The listing builds one solid part. Answer for the finished solid, in the listing's coordinates (mm). A direction names the side the tool comes from. Round coordinates to 2 decimals unless told otherwise and drop trailing zeros. Write each loop counter-clockwise with the first axis right and the second up, starting at its lowest first coordinate (ties: lowest second). Pieces come first, ordered by that corner, then holes. Notation, with made-up numbers: (58, 41.25) - (117, 41.25) arc R9 cw to (117, 45.25) - close; hole circle Ø11 at (-38, 52.5). An arc over 180 degrees is marked (long way). Use a Markdown table: item, result. Add a question column.
1) Find the intervals of material crossed by probe 1 along X at (y, z) = (16.5, 0); probe 2 along Z at (x, y) = (0, 8); probe 3 along X at (y, z) = (-1, -7.5), in increasing order. Write a range as from..to.
2) A tool of negligible diameter and unlimited length cuts with its end or side. For faces 5 (the cylindrical face through (-74.77, -2.43, 0.08)), 6 (the flat face through (28, 50, 0)), 7 (the cylindrical face through (-3.905, 11.739, -0.867)), 8 (the flat face through (26, -5, 0)), 9 (the flat face through (1, -9.529, 0)), from which of +Z, -Z, +X, -X, +Y, -Y can it reach the whole face along a straight path? Write none if from no direction.
3) A cutting plane is placed at D-D (z = 0). State how many separate pieces and enclosed holes the cut face has, then the cut area to 3 significant figures.
4) Each of these flat-tipped pins is pushed along its axis until it touches: P1, Ø9, axis at x = -0.5, z = -1, coming from the +Y side; P2, Ø23, axis at x = 82.5, z = 11, coming from the +Y side; P3, Ø2, axis at x = 25, z = 5.5, coming from the +Y side. Where does it stop, or does it pass through?
5) A cutting plane is placed at C-C (y = 28.5). Give the vertices of the cut face in (x, z).
6) A cutting plane is placed at B-B (y = 9.5). Give the vertices of the cut face in (x, z).
7) A cutting plane is placed at A-A (x = -39). Give the vertices of the cut face in (y, z), then the cut area to 3 significant figures.
8) Determine the mould class of faces 1 (the flat face through (1, 17, -23)), 2 (the cylindrical face through (-90.474, -2.431, -0.087)), 3 (the cylindrical face through (-44.857, 29.877, -1.301)), 4 (the flat face through (-102.03, -2.63, 0.32)) for opening direction X: +X half, -X half, draft (parallel to the pull), parting line (faces both ways), or undercut.
```python
from build123d import *

# Parameters (mm, degrees)
BOSS_EXTRUDE1_DEPTH = 23
SKETCH2_R           = 6
CUT_EXTRUDE1_DEPTH  = 127.368508735
CUT_EXTRUDE2_DEPTH  = 54
CUT_EXTRUDE3_DEPTH  = 120.419428905
SKETCH5_R           = 4
CUT_EXTRUDE18_DEPTH = 24
SKETCH6_W           = 26
SKETCH6_H           = 26
CUT_EXTRUDE19_DEPTH = 10


with BuildPart() as part:
    # Sketch1 → Boss-Extrude1 (new, symmetric)
    with BuildSketch(Plane.XY):
        with BuildLine():
            Line((100, 4.470588235), (104, -9.529411765))
            Line((104, -9.529411765), (-104, -9.529411765))
            Line((-104, -9.529411765), (-100, 4.470588235))
            Line((-100, 4.470588235), (-54, 4.470588235))
            Line((-54, 4.470588235), (-54, 58.470588235))
            Line((-54, 58.470588235), (-28, 58.470588235))
            Line((-28, 58.470588235), (-28, 42.470588235))
            Line((-28, 42.470588235), (-24, 42.470588235))
            ThreePointArc((-24, 42.470588235), (0, 18.470588235), (24, 42.470588235))
            Line((24, 42.470588235), (28, 42.470588235))
            Line((28, 42.470588235), (28, 58.470588235))
            Line((28, 58.470588235), (54, 58.470588235))
            Line((54, 58.470588235), (54, 4.470588235))
            Line((54, 4.470588235), (100, 4.470588235))
        make_face()
    extrude(amount=BOSS_EXTRUDE1_DEPTH, both=True)

    # Sketch2 → Cut-Extrude1 (cut, through all)
    with BuildSketch(Plane(origin=(0, 58.470588235, 0), x_dir=(1, 0, 0), z_dir=(0, 1, 0))):
        with Locations(Location((-39, 0, 0), (0, 0, 270))):
            Circle(SKETCH2_R)
        with Locations(Location((39, 0, 0), (0, 0, 270))):
            Circle(SKETCH2_R)
    extrude(amount=-CUT_EXTRUDE1_DEPTH, mode=Mode.SUBTRACT)

    # Sketch3 → Cut-Extrude2 (cut)
    with BuildSketch(Plane(origin=(0, 58.470588235, 0), x_dir=(1, 0, 0), z_dir=(0, 1, 0))):
        with BuildLine():
            Line((-48.856934001, 23), (-69.801648505, 23))
            Line((-69.801648505, 23), (-69.801648505, -23))
            Line((-69.801648505, -23), (-48.856934001, -23))
            ThreePointArc((-48.856934001, -23), (-54, 0), (-48.856934001, 23))
        make_face()
        with BuildLine():
            Line((69.801648505, -23), (48.856934001, -23))
            ThreePointArc((48.856934001, -23), (54, 0), (48.856934001, 23))
            Line((48.856934001, 23), (69.801648505, 23))
            Line((69.801648505, 23), (69.801648505, -23))
        make_face()
    extrude(amount=-CUT_EXTRUDE2_DEPTH, mode=Mode.SUBTRACT)

    # Sketch4 → Cut-Extrude3 (cut, through all)
    with BuildSketch(Plane(origin=(0, 4.470588235, 0), x_dir=(1, 0, 0), z_dir=(0, 1, 0))):
        with BuildLine():
            Line((-86.259028478, 3.967568831), (-86.5, 3.974879835))
            ThreePointArc((-86.5, 3.974879835), (-90.474879835, 0), (-86.5, -3.974879835))
            Line((-86.5, -3.974879835), (-86.259028478, -3.967568831))
            Line((-86.259028478, -3.967568831), (-78.5, -3.732162222))
            ThreePointArc((-78.5, -3.732162222), (-74.767837778, 0), (-78.5, 3.732162222))
            Line((-78.5, 3.732162222), (-86.259028478, 3.967568831))
        make_face()
    cut_extrude3 = extrude(amount=-CUT_EXTRUDE3_DEPTH, mode=Mode.SUBTRACT)

    # Mirror1: Cut-Extrude3 across plane
    add(cut_extrude3.mirror(Plane(origin=(0, 0, 0), x_dir=(0, 0, 1), z_dir=(1, 0, 0))), mode=Mode.SUBTRACT)

    # Sketch5 → Cut-Extrude18 (cut)
    with BuildSketch(Plane(origin=(0, 28.470588235, 0), x_dir=(1, 0, 0), z_dir=(0, 1, 0))):
        with Locations(Location((0, 0, 0), (0, 0, 270))):
            Circle(SKETCH5_R)
    extrude(amount=-CUT_EXTRUDE18_DEPTH, mode=Mode.SUBTRACT)

    # Sketch6 → Cut-Extrude19 (cut)
    with BuildSketch(Plane.XZ.offset(9.529411765)):
        with Locations((-39, 0)):
            Rectangle(SKETCH6_W, SKETCH6_H)
        with Locations((39, 0)):
            Rectangle(SKETCH6_W, SKETCH6_H)
    extrude(amount=-CUT_EXTRUDE19_DEPTH, mode=Mode.SUBTRACT)


solid = part.part
```
Entries:
| question | item | result |
|---|---|---|
| 1 | probe 1 | x = -54..-45, -33..-4, 4..33, 45..54 |
| 1 | probe 2 | z = -23..-4, 4..23 |
| 1 | probe 3 | x = -101.56..-52, -26..26, 52..101.56 |
| 2 | face 5 | +Y, -Y |
| 2 | face 6 | +Z, -Z, +Y |
| 2 | face 7 | +Y |
| 2 | face 8 | -Y |
| 2 | face 9 | +Z, -Z, +X, -X, -Y |
| 3 | separate pieces | 5 |
| 3 | enclosed holes | 0 |
| 3 | area | 4,420 mm² |
| 4 | P1 | stops at y = 19 |
| 4 | P2 | stops at y = 4.47 |
| 4 | P3 | stops at y = 42.47 |
| 5 | outline | (-48.86, -23) - (-19.51, -23) - (-19.51, 23) - (-48.86, 23) arc R54 ccw to start; (19.51, -23) - (48.86, -23) arc R54 ccw to (48.86, 23) - (19.51, 23) - close; hole circle Ø12 at (-39, 0); hole circle Ø12 at (39, 0) |
| 6 | outline | (-48.86, -23) - (48.86, -23) arc R54 ccw to (48.86, 23) - (-48.86, 23) arc R54 ccw to start; hole circle Ø12 at (-39, 0); hole circle Ø8 at (0, 0); hole circle Ø12 at (39, 0) |
| 7 | outline | (-9.53, -23) - (58.47, -23) - (58.47, -6) - (0.47, -6) - (0.47, -13) - (-9.53, -13) - close; (-9.53, 13) - (0.47, 13) - (0.47, 6) - (58.47, 6) - (58.47, 23) - (-9.53, 23) - close |
| 7 | area | 2,170 mm² |
| 8 | face 1 | draft |
| 8 | face 2 | undercut |
| 8 | face 3 | undercut |
| 8 | face 4 | -X half |
